Autodesk Inventor part; units mm, degrees
ref_plane "Feeder Plane" through (0, 0, -10) normal (1, 0, 0) x (0, 0, 1)
ref_plane "Feeder Work Plane" through (0, 0, 1300) normal (0, -1, 0) x (1, 0, 0)
ref_plane "Inner Plane" through (0, 0, 0) normal (0.7071, 0.7071, 0) x (-0.7071, 0.7071, 0)
sketch "Sketch1" plane through (0, 0, 0) normal (0, 1, 0) x (-1, 0, 0)
  line L0 (476, 1500) -> (470, 1500)
  line L1 (470, 1500) -> (470, 0)
  line L2 (470, 0) -> (476, 0)
  line L3 (476, 0) -> (476, 1500)
  line L4 (0, 0) -> (0, 1673.0415)
  point P0 (473, 0)
  dimension "d0" = 6
  dimension "d1" = 1500
  dimension "d2" = 940
revolve "Revolution1" add sketch "Sketch1" angle 359.9 about axis through (0, 0, 0) along (0, 0, 1)
sketch "Sketch2" plane through (0, 0, 0) normal (0, 1, 0) x (-1, 0, 0)
  circle A0 centre (0, 400) radius 267.5
  line L0 (470, 1500) -> (-470, 1500)
  line L1 (110, 1300) -> (-110, 1300) construction
  line L2 (110, 1390) -> (-110, 1390)
  line L3 (-110, 1210) -> (110, 1210)
  arc A1 (110, 1210) -> (110, 1390) centre (110, 1300) ccw
  arc A2 (-110, 1390) -> (-110, 1210) centre (-110, 1300) ccw
  line L4 (200, 1300) -> (-200, 1300) construction
  point P0 (0, 0)
  point P1 (469.9993, 1500)
  point P2 (0, 1300)
  dimension "d4" = 535
  dimension "d12" = 400
  dimension "d15" = 200
  dimension "d16" = 400
  dimension "d17" = 180
extrude "Extrusion1" cut sketch "Sketch2" against normal through all contours A0
sketch "floor angle sketch" plane through (0, 0, 0) normal (0, 0, 1) x (1, 0, 0)
  line L0 (0, 0) -> (0, -267.717)
  line L1 (0, -267.717) -> (0, 0)
  line L2 (0, 0) -> (0, -172)
  line L3 (0, 0) -> (-63.6396, 63.6396)
  line L4 (0, 0) -> (23.2937, -86.9333)
  dimension "Feeder_way_angle" = 0
  dimension "Feeder_way_line" = 172
  dimension "Outer_way_line" = 90
  dimension "Inner_way_line" = 90
  dimension "Outer_way_angle" = 345
  dimension "Inner_way_angle" = 135
ref_plane "Feeder Plane" through (0, 0, -10) normal (1, 0, 0) x (0, 0, 1)
sketch "Feeder horisont hight angle" plane through (0, 0, -10) normal (1, 0, 0) x (0, 0, 1)
  line L0 (1510, -470) -> (1510, 470) construction
  line L1 (10, 0) -> (1510, 0) construction
  line L2 (1310, 0) -> (1310, 476)
  line L3 (10, 476) -> (1510, 476) construction
  line L4 (1310, 476) -> (1310, 0) construction
  point P0 (1510, 0)
  point P1 (1510, -0.8203)
  dimension "d34" = 1300
  dimension "d35" = 0
ref_plane "Feeder Work Plane" through (0, 0, 1300) normal (0, -1, 0) x (1, 0, 0)
sketch "Sketch8" plane through (0, 0, 1300) normal (0, -1, 0) x (1, 0, 0)
  circle A0 centre (0, 0) radius 86 construction
  line L0 (-100, 50) -> (100, 50)
  line L1 (100, 50) -> (100, -50)
  line L2 (100, -50) -> (-100, -50)
  line L3 (-100, -50) -> (-100, 50)
  line L4 (-100, 50) -> (100, -50) construction
  line L5 (100, 50) -> (-100, -50) construction
  arc A1 (-100, -50) -> (100, -50) centre (0, 409.2385) ccw construction
  arc A2 (-100, 50) -> (100, 50) centre (0, 509.2385) ccw construction
  point P0 (0, -1300)
  point P1 (0, 0)
  dimension "d36" = 172
  dimension "d50" = 200
  dimension "d51" = 100
  dimension "d52" = 470
extrude "Feeder Extrusion" cut sketch "Sketch8" along normal through all
ref_plane "Inner Plane" through (0, 0, 0) normal (0.7071, 0.7071, 0) x (-0.7071, 0.7071, 0)
sketch "Inner horisont hight angle" plane through (0, 0, 0) normal (0.7071, 0.7071, 0) x (-0.7071, 0.7071, 0)
  line L0 (476, 1500) -> (-476, 1500) construction
  line L1 (476, 0) -> (476, 1500) construction
  line L2 (0, 0) -> (0, 1500) construction
  line L3 (0, 1200) -> (476, 1200) construction
  line L4 (476, 1200) -> (0, 1200)
  point P0 (336.5828, 1500)
  point P1 (337.1698, 1500)
  dimension "d40" = 0
  dimension "d41" = 1200
ref_plane "Inner Work Plane" through (0, 0, 1200) normal (0.7071, -0.7071, 0) x (0.7071, 0.7071, 0)
sketch "Sketch10" plane through (0, 0, 1200) normal (0.7071, -0.7071, 0) x (0.7071, 0.7071, 0)
  circle A0 centre (0, 0) radius 45.5
  point P0 (0, -1200)
  point P1 (0, 0)
  point P2 (0, 0)
  point P3 (0, 0)
  dimension "d42" = 91
extrude "Inner Extrusion" cut sketch "Sketch10" against normal through all
ref_plane "Outer Plane" through (0, 0, 0) normal (-0.9659, -0.2588, 0) x (0.2588, -0.9659, 0)
sketch "Sketch11" plane through (0, 0, 0) normal (-0.9659, -0.2588, 0) x (0.2588, -0.9659, 0)
  line L0 (0, 0) -> (0, 1500)
  line L1 (476, 1500) -> (-476, 1500)
  line L2 (0, 700) -> (476, 700)
  line L3 (476, 0) -> (476, 1500)
  line L4 (476, 700) -> (0, 700)
  point P0 (-123.1979, 1500)
  point P1 (-124.0001, 1500)
  dimension "d45" = 0
  dimension "d46" = 700
ref_plane "Work Plane9" through (0, 0, 700) normal (-0.2588, 0.9659, 0) x (-0.9659, -0.2588, 0)
sketch "Sketch12" plane through (0, 0, 700) normal (-0.2588, 0.9659, 0) x (-0.9659, -0.2588, 0)
  circle A0 centre (0, 0) radius 46
  point P0 (0, -700)
  point P1 (0, 0)
  point P2 (0, 0)
  point P3 (0, 0)
  dimension "d47" = 92
extrude "Extrusion6" [suppressed]
equation "\"d2\" = MAIN_filter_diam"
equation "\"d4\" = Accsess_hatch_diameter"
equation "\"d16\" = Charging_hatch_width"
equation "\"d17\" = Charging_hatch_hight"
equation "\"d34\" = Feedr_hight"
equation "\"BendRadius\" = Thickness"
equation "\"BendReliefWidth\" = Thickness"
equation "\"BendReliefDepth\" = 0.5 * Thickness"
equation "\"CornerReliefSize\" = 4 * Thickness"
equation "\"MinimumRemnant\" = 2 * Thickness"
equation "\"TransitionRadius\" = BendRadius"
equation "\"JacobiRadiusSize\" = BendRadius"
equation "\"GapSize\" = Thickness"
equation "\"Feedr_hight\" = 1300"
equation "\"Feeder_horisont_hight_angle\" = 0"
equation "\"MAIN_filter_diam\" = 940"
equation "\"Accsess_hatch_diameter\" = 535"
equation "\"Charging_hatch_width\" = 400"
equation "\"Charging_hatch_hight\" = 180"
properties part number "SLM 701 main shell D1200" material "Steel"
Check sheet for the modelled part. Datum: model origin and axes. Units: mm. A direction names the side the tool comes from. Round coordinates to 2 decimals unless told otherwise and drop trailing zeros. Loops run counter-clockwise (first coordinate to the right, second up) from the corner with the lowest first, then second, coordinate; pieces in that order, holes last. Notation, with made-up numbers: (-10, -34) - (18, -34) arc R12 cw to (18, -26) - close; hole circle Ø9 at (0, 73). An arc over 180 degrees is marked (long way). Answer as CSV lines item,"result". Start each with the question number.
Item 1: Set-up check for faces 1 (the cylindrical face through (207.42, -427.7, 231.08)), 2 (the cylindrical face through (-359.17, 308.11, 1172.31)): record each of +Z, -Z, +X, -X, +Y, -Y from which the full face is reachable in a straight line by a thin tool's end or side.
Item 2: Section check B-B (x = 0). Record the boundary of the cut face in (y, z), and give its area (3 significant figures).
Item 3: Section check A-A (z = 554.5). Record the boundary of the cut face in (x, y), and give its area (3 significant figures).
Item 4: Scan lines: line 1 (Y direction, x = -16, z = 920); line 2 (Y direction, x = 0, z = 1139); line 3 (X direction, y = 336.5, z = 1426.5). Record each from-to range of solid material in increasing order. Write a range as [from, to].
Item 5: Depth check by flat-ended pin: P1, Ø2, axis at y = -15.5, z = 1263.5, coming from the +X side; P2, Ø3, axis at x = 65.5, z = 987, coming from the -Y side; P3, Ø1.5, axis at x = 33, z = 724.5, coming from the +Y side. Enter the tip coordinate at first touch or a pass-through.
Item 6: Section check C-C (y = 22.5). Record the boundary of the cut face in (x, z), and give its area (3 significant figures).
Item 7: Release check for a two-part mould opening along Y. For faces 3 (the cylindrical face through (103.77, 464.55, 760.5)), 4 (the cylindrical face through (61.78, 465.92, 739.5)), 5 (the flat face through (-350, 315, 1500)) record: +Y half, -Y half, draft (parallel to the pull), parting line (faces both ways), or undercut.
Item 8: Section check D-D (z = 1403.5). Record the boundary of the cut face in (x, y), and give its area (3 significant figures).
Report:
1,face 1,"-Y"
1,face 2,"none"
2,outline,"(-476, 0) - (-470, 0) - (-470, 132.5) - (-476, 132.5) - close; (-476, 667.5) - (-470, 667.5) - (-470, 1250) - (-476, 1250) - close; (-476, 1350) - (-470, 1350) - (-470, 1500) - (-476, 1500) - close; (470, 0) - (476, 0) - (476, 1500) - (470, 1500) - close"
2,area,"14,200 mm2"
3,outline,"(-476, 0) arc R476 ccw to (-218.37, -422.95) - (-218.37, -416.19) arc R470 cw to (-470, 0) - close; (-476, 0.83) - (-470, 0.82) arc R470 cw (long way) to (218.37, -416.19) - (218.37, -422.95) arc R476 ccw (long way) to start"
3,area,"15,100 mm2"
4,line 1,"y = [-475.73, -469.73], [469.73, 475.73]"
4,line 2,"y = [-476, -470], [470, 476]"
4,line 3,"x = [-336.67, -328.13], [328.13, 336.67]"
5,P1,"stops at x = 475.78"
5,P2,"stops at y = -471.68"
5,P3,"stops at y = 474.91"
6,outline,"(-475.47, 0) - (-469.46, 0) - (-469.46, 1500) - (-475.47, 1500) - close; (469.46, 0) - (475.47, 0) - (475.47, 1500) - (469.46, 1500) - close"
6,area,"18,000 mm2"
7,face 3,"parting line"
7,face 4,"undercut"
7,face 5,"draft"
8,outline,"(-476, 0) arc R476 ccw (long way) to (-476, 0.83) - (-470, 0.82) arc R470 cw (long way) to (-470, 0) - close"
8,area,"17,800 mm2"
